Here's how the part is built. I have some questions about the finished solid (model axes, mm). A direction names the side the tool comes from. Round coordinates to 2 decimals unless told otherwise and drop trailing zeros. Write each loop counter-clockwise with the first axis right and the second up, starting at its lowest first coordinate (ties: lowest second). Pieces come first, ordered by that corner, then holes. Notation, with made-up numbers: (52.5, 29.5) -> (104.5, 29.5) arc R28 cw to (104.5, 62.5) -> close; hole circle Ø6 at (-24, 42.5). An arc over 180 degrees is marked (long way). Put each result on its own line as item: value. Start each with the question number.
1) Which directions (+Z, -Z, +X, -X, +Y, -Y) give clear straight access to the entire face, cutting with the end or side of a thin tool? Please do faces 1 (the flat face through (25, -3.46, -18)), 2 (the cylindrical face through (-22.117, -0.066, -17.853)), 3 (the flat face through (0, 3, -3.175)).
2) I want a section at C-C, the plane y = 0. List the corners of the cut face in (x, z) for me (3 decimals).
3) I want a section at A-A, the plane x = -23.5. List the corners of the cut face in (y, z) for me, then the cut area to 3 significant figures.
4) Will these pins go through, and if not, where does the flat tip stop? P1, Ø8, axis at x = 18, z = -18, coming from the +Y side; P2, Ø5, axis at y = 0, z = -33, coming from the -X side; P3, Ø3.5, axis at y = 1.5, z = -20.5, coming from the -X side.
5) If I drill on line 1 along X through (y, z) = (2, -9); line 2 along X through (y, z) = (5, -33); line 3 along Y through (x, z) = (0, -1.65), over which ranges is the centre line in solid material (lowest first)? Write a range as [from, to].
6) I want a section at B-B, the plane z = -7.5. List the corners of the cut face in (x, y) for me, then the cut area to 3 significant figures.
7) We'd pull the mould along Y, two halves only. Please class faces 4 (the flat face through (21.784, 1.4, -27.7)), 5 (the flat face through (-24, -5, -37.211)), 6 (the flat face through (6, -6, -2)): released by +Y, released by -Y, zero draft, split by the parting line, or undercut.
8) I want a section at D-D, the plane z = -33. Give the number of separate pieces and of enclosed holes in the cut face, then the cut area to 3 significant figures.
from build123d import *

# Parameters (mm, degrees)
SKETCH1_W           = 42.04380551
SKETCH1_H           = 12
SKETCH1_R           = 2.754
BOSS_EXTRUDE1_DEPTH = 3.175
BOSS_EXTRUDE2_DEPTH = 37.211
CUT_EXTRUDE1_DEPTH  = 63.479858345
CUT_EXTRUDE2_DEPTH  = 0.67464881
CUT_EXTRUDE3_START  = -0.67464881
CUT_EXTRUDE3_DEPTH  = 0.67464881
FILLET1_R           = 2.54
CUT_EXTRUDE4_DEPTH  = 9.906
BOSS_EXTRUDE3_DEPTH = 0.762
BOSS_EXTRUDE4_START = -0.762
BOSS_EXTRUDE4_DEPTH = 0.762


with BuildPart() as part:
    # Sketch1 → Boss-Extrude1 (new body)
    with BuildSketch(Plane.XY):
        Rectangle(SKETCH1_W, SKETCH1_H)
        Circle(SKETCH1_R, mode=Mode.SUBTRACT)
    extrude(amount=-BOSS_EXTRUDE1_DEPTH)

    # Sketch2 → Boss-Extrude2 (add)
    with BuildSketch(Plane.XY):
        Polygon((27.371902755, 3.46), (27.371902755, 6), (21.021902755, 6), (21.021902755, -6), (27.371902755, -6), (27.371902755, -3.46), (22.458551565, -3.46), (22.458551565, 3.46), align=None)
    boss_extrude2 = extrude(amount=-BOSS_EXTRUDE2_DEPTH)

    # Mirror1: Boss-Extrude2 across plane
    add(boss_extrude2.mirror(Plane(origin=(0, 0, 0), x_dir=(0, 0, 1), z_dir=(1, 0, 0))))

    # Sketch3 → Cut-Extrude1 (cut, through all)
    with BuildSketch(Plane(origin=(22.458551565, 0, 0), x_dir=(0, 0, -1), z_dir=(1, 0, 0))):
        with BuildLine():
            Line((31.771902755, 1.75), (20.871902755, 1.75))
            ThreePointArc((20.871902755, 1.75), (19.121902755, 0), (20.871902755, -1.75))
            Line((20.871902755, -1.75), (31.771902755, -1.75))
            ThreePointArc((31.771902755, -1.75), (33.521902755, 0), (31.771902755, 1.75))
        make_face()
    extrude(amount=-CUT_EXTRUDE1_DEPTH, mode=Mode.SUBTRACT)

    # Sketch4 → Cut-Extrude2 (cut)
    with BuildSketch(Plane(origin=(22.458551565, 0, 0), x_dir=(0, 0, -1), z_dir=(1, 0, 0))):
        with BuildLine():
            Line((31.771902755, 3.02), (20.871902755, 3.02))
            ThreePointArc((20.871902755, 3.02), (17.851902755, 0), (20.871902755, -3.02))
            Line((20.871902755, -3.02), (31.771902755, -3.02))
            ThreePointArc((31.771902755, -3.02), (34.791902755, 0), (31.771902755, 3.02))
        make_face()
    extrude(amount=-CUT_EXTRUDE2_DEPTH, mode=Mode.SUBTRACT)

    # Sketch5 → Cut-Extrude3 (cut)
    with BuildSketch(Plane.ZY.offset(22.458551565).offset(CUT_EXTRUDE3_START)):
        with BuildLine():
            Line((-20.871902755, 3.02), (-31.771902755, 3.02))
            ThreePointArc((-31.771902755, 3.02), (-34.791902755, 0), (-31.771902755, -3.02))
            Line((-31.771902755, -3.02), (-20.871902755, -3.02))
            ThreePointArc((-20.871902755, -3.02), (-17.851902755, 0), (-20.871902755, 3.02))
        make_face()
    extrude(amount=CUT_EXTRUDE3_DEPTH, mode=Mode.SUBTRACT)

    # Fillet1
    fillet1_edges = [part.edges().sort_by_distance(p)[0] for p in [
        (-21.021902755, 0, -3.175),
        (21.021902755, 0, -3.175),
    ]]
    fillet(fillet1_edges, radius=FILLET1_R)

    # Sketch6 → Cut-Extrude4 (cut)
    with BuildSketch(Plane(origin=(0, 0, -37.211), x_dir=(-1, 0, 0), z_dir=(0, 0, -1))):
        Polygon((-21.783902755, -3.02), (-22.458551565, -3.02), (-22.458551565, 3.02), (-21.783902755, 3.02), (-21.783902755, 1.75), (-21.021902755, 1.75), (-21.021902755, -1.75), (-21.783902755, -1.75), align=None)
    cut_extrude4 = extrude(amount=-CUT_EXTRUDE4_DEPTH, mode=Mode.SUBTRACT)

    # Mirror2: Cut-Extrude4 across plane
    add(cut_extrude4.mirror(Plane(origin=(0, 0, 0), x_dir=(0, 0, 1), z_dir=(1, 0, 0))), mode=Mode.SUBTRACT)

    # Sketch8 → Boss-Extrude3 (add)
    with BuildSketch(Plane(origin=(-21.021902755, 0, 0), x_dir=(0, 0, -1), z_dir=(1, 0, 0))):
        with BuildLine():
            Line((20.871902755, 0.861), (37.211, 0.861))
            Line((37.211, 0.861), (37.211, 1.75))
            Line((37.211, 1.75), (20.871902755, 1.75))
            ThreePointArc((20.871902755, 1.75), (19.121902755, 0), (20.871902755, -1.75))
            Line((20.871902755, -1.75), (37.211, -1.75))
            Line((37.211, -1.75), (37.211, -0.861))
            Line((37.211, -0.861), (20.871902755, -0.861))
            ThreePointArc((20.871902755, -0.861), (20.010902755, 0), (20.871902755, 0.861))
        make_face()
    extrude(amount=-BOSS_EXTRUDE3_DEPTH)

    # Sketch9 → Boss-Extrude4 (add)
    with BuildSketch(Plane.ZY.offset(-21.021902755).offset(BOSS_EXTRUDE4_START)):
        with BuildLine():
            Line((-20.871902755, -3.02), (-37.211, -3.02))
            Line((-37.211, -3.02), (-37.211, -0.861))
            Line((-37.211, -0.861), (-20.871902755, -0.861))
            ThreePointArc((-20.871902755, -0.861), (-20.010902755, 0), (-20.871902755, 0.861))
            Line((-20.871902755, 0.861), (-37.211, 0.861))
            Line((-37.211, 0.861), (-37.211, 3.02))
            Line((-37.211, 3.02), (-20.871902755, 3.02))
            ThreePointArc((-20.871902755, 3.02), (-17.851902755, 0), (-20.871902755, -3.02))
        make_face()
    extrude(amount=BOSS_EXTRUDE4_DEPTH)


solid = part.part
Findings:
1. face 1: +Z, -Z, +X
1. face 2: -Z, -X
1. face 3: -Z, +Y, -Y
2. outline: (-22.459, -17.852) -> (-21.784, -17.852) -> (-21.784, -20.011) -> (-21.022, -20.011) -> (-21.022, -5.715) arc R2.54 cw to (-18.482, -3.175) -> (-2.754, -3.175) -> (-2.754, 0) -> (-22.459, 0) -> close; (2.754, -3.175) -> (18.482, -3.175) arc R2.54 cw to (21.022, -5.715) -> (21.022, -20.011) -> (21.784, -20.011) -> (21.784, -17.852) -> (22.459, -17.852) -> (22.459, 0) -> (2.754, 0) -> close
3. outline: (-6, -37.21) -> (-3.46, -37.21) -> (-3.46, 0) -> (-6, 0) -> close; (3.46, -37.21) -> (6, -37.21) -> (6, 0) -> (3.46, 0) -> close
3. area: 189 mm2
4. P1: stops at y = 6
4. P2: stops at x = -21.78
4. P3: stops at x = -22.46
5. line 1: x = [-22.46, -21.02], [21.02, 22.46]
5. line 2: x = [-27.37, -21.02], [21.02, 27.37]
5. line 3: y = [-6, -2.75], [2.75, 6]
6. outline: (-27.37, -6) -> (-21.02, -6) -> (-21.02, 6) -> (-27.37, 6) -> (-27.37, 3.46) -> (-22.46, 3.46) -> (-22.46, -3.46) -> (-27.37, -3.46) -> close; (21.02, -6) -> (27.37, -6) -> (27.37, -3.46) -> (22.46, -3.46) -> (22.46, 3.46) -> (27.37, 3.46) -> (27.37, 6) -> (21.02, 6) -> close
6. area: 84.4 mm2
7. face 4: undercut
7. face 5: zero draft
7. face 6: released by -Y
8. separate pieces: 4
8. enclosed holes: 0
8. area: 73.6 mm2
